Can you work these out from the model? Positions are in its coordinate system, mm. Give positions to 0.01 mm unless a question says otherwise; leave off trailing zeros. Loops run counter-clockwise (first coordinate to the right, second up) from the corner with the lowest first, then second, coordinate; pieces in that order, holes last. Notation, with made-up numbers: M 48.5,50 L 56.5,50 A28 cw 56.5,70 Z; hole C 27,35.25 d10. An arc over 180 degrees is marked long. Put each result on its own line as item: value. Start each with the question number.
1) Please list where these lines run through material, in increasing order: line 1 along X through (y, z) = (-4, -13.5); line 2 along Y through (x, z) = (-90, -1.1); line 3 along X through (y, z) = (5, -44.5). Write a range as from..to.
2) For P1, Ø4.5, axis at x = 90, y = 0, coming from the -Z side; P2, Ø6.5, axis at x = 91, y = 1.5, coming from the +Z side; P3, Ø5, axis at x = -157.31, z = -13.5, coming from the +Y side, each with a flat end and sliding along its axis, tell me the tip position at first contact or that it passes through.
3) Imagine slicing it at B-B (x = -6.5). Write out the boundary of the cut face in (y, z).
4) Imagine slicing it at A-A (z = -55). Write out the boundary of the cut face in (x, y), then the cut area to 3 significant figures.
from build123d import *

# Parameters (mm, degrees)
SKETCH1_W                                        = 296.88
SKETCH1_H                                        = 15
BOSS_EXTRUDE1_DEPTH                              = 10
CBORE_FOR_M3_HEX_HEAD_MACHINE_SCREW1_D           = 3.4
CBORE_FOR_M3_HEX_HEAD_MACHINE_SCREW1_CBORE_D     = 8.4
CBORE_FOR_M3_HEX_HEAD_MACHINE_SCREW1_CBORE_DEPTH = 2.3
SKETCH5_W                                        = 40
SKETCH5_H                                        = 90
BOSS_EXTRUDE2_DEPTH                              = 15
CBORE_FOR_M4_HEX_HEAD_MACHINE_SCREW1_D           = 4.5
CBORE_FOR_M4_HEX_HEAD_MACHINE_SCREW1_CBORE_D     = 10.59
CBORE_FOR_M4_HEX_HEAD_MACHINE_SCREW1_CBORE_DEPTH = 3
BOSS_EXTRUDE3_DEPTH                              = 15
SKETCH13_W                                       = 368.635882897
SKETCH13_H                                       = 90
BOSS_EXTRUDE4_DEPTH                              = 15
M4_CLEARANCE_HOLE1_D                             = 4.5
M4X0_7_TAPPED_HOLE1_D                            = 3.3
M4X0_7_TAPPED_HOLE1_DEPTH                        = 10.1
M4X0_7_TAPPED_HOLE1_TIP                          = 0.991420021


with BuildPart() as part:
    # Sketch1 → Boss-Extrude1 (new body)
    with BuildSketch(Plane.XY):
        Rectangle(SKETCH1_W, SKETCH1_H)
    extrude(amount=-BOSS_EXTRUDE1_DEPTH)

    # CBORE for M3 Hex Head Machine Screw1 (through all)
    with Locations(Plane.XY):
        with Locations((-90, 0), (90, 0)):
            CounterBoreHole(CBORE_FOR_M3_HEX_HEAD_MACHINE_SCREW1_D / 2, CBORE_FOR_M3_HEX_HEAD_MACHINE_SCREW1_CBORE_D / 2, CBORE_FOR_M3_HEX_HEAD_MACHINE_SCREW1_CBORE_DEPTH)

    # Sketch5 → Boss-Extrude2 (add)
    with BuildSketch(Plane(origin=(0, 7.5, 0), x_dir=(1, 0, 0), z_dir=(0, 1, 0))):
        with Locations((-168.44, 45)):
            Rectangle(SKETCH5_W, SKETCH5_H)
    extrude(amount=-BOSS_EXTRUDE2_DEPTH)

    # CBORE for M4 Hex Head Machine Screw1 (through all)
    with Locations(Plane(origin=(0, 7.5, 0), x_dir=(1, 0, 0), z_dir=(0, 1, 0))):
        with Locations((-177.311326024, 13.5), (-157.311326024, 13.5), (-177.311326024, 78.5), (-157.311326024, 78.5)):
            CounterBoreHole(CBORE_FOR_M4_HEX_HEAD_MACHINE_SCREW1_D / 2, CBORE_FOR_M4_HEX_HEAD_MACHINE_SCREW1_CBORE_D / 2, CBORE_FOR_M4_HEX_HEAD_MACHINE_SCREW1_CBORE_DEPTH)

    # Sketch12 → Boss-Extrude3 (add)
    with BuildSketch(Plane(origin=(0, 7.5, 0), x_dir=(1, 0, 0), z_dir=(0, 1, 0))):
        Polygon((-188.44, 0), (-178.44, -10), (-148.44, -10), (-120.965225805, 0), align=None)
    extrude(amount=-BOSS_EXTRUDE3_DEPTH)

    # Sketch13 → Boss-Extrude4 (add)
    with BuildSketch(Plane(origin=(0, 7.5, 0), x_dir=(1, 0, 0), z_dir=(0, 1, 0))):
        with Locations((-372.757941448, 45)):
            Rectangle(SKETCH13_W, SKETCH13_H)
    extrude(amount=-BOSS_EXTRUDE4_DEPTH)

    # M4 Clearance Hole1 (through all)
    with Locations(Plane(origin=(0, 7.5, 0), x_dir=(1, 0, 0), z_dir=(0, 1, 0))):
        with Locations((-547.075882897, 78.5), (-527.075882897, 78.5), (-527.075882897, 13.5), (-547.075882897, 13.5)):
            Hole(M4_CLEARANCE_HOLE1_D / 2)

    # M4x0.7 Tapped Hole1
    with Locations(Plane(origin=(0, 7.5, 0), x_dir=(1, 0, 0), z_dir=(0, 1, 0))):
        with Locations((-507.075882897, 78.5), (-507.075882897, 13.5), (-447.075882897, 13.5), (-427.075882897, 13.5), (-407.075882897, 13.5), (-407.075882897, 78.5), (-427.075882897, 78.5), (-447.075882897, 78.5)):
            Hole(M4X0_7_TAPPED_HOLE1_D / 2, depth=M4X0_7_TAPPED_HOLE1_DEPTH)
            with Locations((0, 0, -(M4X0_7_TAPPED_HOLE1_DEPTH + M4X0_7_TAPPED_HOLE1_TIP / 2))):  # 118° drill point
                Cone(0, M4X0_7_TAPPED_HOLE1_D / 2, M4X0_7_TAPPED_HOLE1_TIP, mode=Mode.SUBTRACT)


solid = part.part
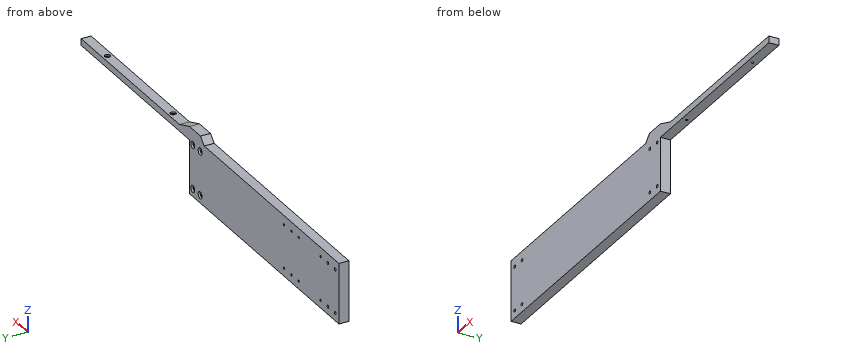
Recorded:
1. line 1: -557.08..-549.33, -544.83..-529.33, -524.83..-179.56, -175.06..-159.56, -155.06..-148.44
1. line 2: -7.5..-4.2, 4.2..7.5
1. line 3: -557.08..-148.44
2. P1: z = -10
2. P2: z = 0
2. P3: y = 4.5
3. outline: M -7.5,-10 L 7.5,-10 L 7.5,0 L -7.5,0 Z
4. outline: M -557.08,-7.5 L -148.44,-7.5 L -148.44,7.5 L -557.08,7.5 Z
4. area: 6,130 mm²
